For this review, take the finished solid that the model builds, in its own axes (mm). A direction names the side the tool comes from. Round coordinates to 2 decimals unless told otherwise and drop trailing zeros. Order: outer loops, then holes, each group sorted by start corner. A loop starts at its lowest first (then second) coordinate and runs counter-clockwise, first axis right, second up. Notation, with made-up numbers: M -21,82 L -7,82 A18 ccw -7,91 Z; hole C -22,15 d1. An arc over 180 degrees is marked long. Answer in a Markdown table with one row per item. Add a question column.
```python
from build123d import *

# Parameters (mm, degrees)
SKETCH_1_W          = 1.5
SKETCH_1_H          = 3
SKETCH_1_W_2        = 3.5
EXTRUDE_1_DEPTH     = 7
SKETCH_2_R          = 1.5
CUT_EXTRUDE_2_DEPTH = 7
SKETCH_4_R          = 1.5
CUT_EXTRUDE_3_DEPTH = 7


with BuildPart() as part:
    # 草图1 → 凸台-拉伸1 (new body)
    with BuildSketch(Plane.XY):
        Polygon((-0.641080243, 21.986723194), (-3.641080243, 21.986723194), (-3.641080243, -9.013276806), (-10.005041274, -15.377237837), (-10.005041274, -31.619878524), (-4.341080243, -31.619878524), (-4.341080243, -28.619878524), (-7.005041274, -28.619878524), (-7.005041274, -16.619878524), (-0.641080243, -10.255917493), align=None)
        with Locations((-2.091080243, -30.119878524)):
            Rectangle(SKETCH_1_W, SKETCH_1_H)
        with Locations((-3.591080243, -30.119878524)):
            Rectangle(SKETCH_1_W, SKETCH_1_H)
        with Locations((0.408919757, -30.119878524)):
            Rectangle(SKETCH_1_W_2, SKETCH_1_H)
    extrude(amount=EXTRUDE_1_DEPTH)

    # 草图2 → 切除-拉伸2 (cut)
    with BuildSketch(Plane.ZY.offset(3.641080243)):
        with Locations(Location((3.5, 18.986723194, 0), (0, 0, 270))):
            Circle(SKETCH_2_R)
        with Locations(Location((3.5, -3.013276806, 0), (0, 0, 270))):
            Circle(SKETCH_2_R)
    extrude(amount=-CUT_EXTRUDE_2_DEPTH, mode=Mode.SUBTRACT)

    # 草图4 → 切除-拉伸3 (cut)
    with BuildSketch(Plane(origin=(0, -28.619878524, 0), x_dir=(1, 0, 0), z_dir=(0, 1, 0))):
        with Locations(Location((-2.841080243, -4, 0), (0, 0, 270))):
            Circle(SKETCH_4_R)
    extrude(amount=-CUT_EXTRUDE_3_DEPTH, mode=Mode.SUBTRACT)


solid = part.part
```
1. The part is to be moulded in two halves that separate along Z. For faces 1 (the cylindrical face through (-3.416, -30.099, 5.386)), 2 (the cylindrical face through (-2.16, -3.71, 2.17)), 3 (the flat face through (-3, -7, 0)), 4 (the flat face through (-10.005, -23, 3)), say which applies: pulls with the +Z half, pulls with the -Z half, needs draft (parallel to the pull), parting line crosses it, or undercut.
2. Clearance check with flat-ended pins moving along their axes: pin 1 Ø1 at (y, z) = (-10, 3) entering from +X; pin 2 Ø2.5 at (y, z) = (-3.01, 3.5) entering from +X; pin 3 Ø2 at (x, z) = (-6, 3.5) entering from +Y. State where each tip first meets the part, or that it passes through.
3. Consider section D-D on x = 0.5. Write out the cut boundary in (y, z).
4. Consider section B-B on x = -2.25. Write out the cut boundary in (y, z), plus the area to 3 significant figures.
5. Consider section C-C on y = 17. Write out the cut boundary in (x, z), plus the area to 3 significant figures.
6. To check wall thickness, follow probe 1 along X at (y, z) = (-30.05, 4); probe 2 along X at (y, z) = (-20.5, 3); probe 3 along Y at (x, z) = (1, 5). State the ranges of each line that lie inside material, in increasing order. Write a range as [from, to].
7. Consider section A-A on z = 3. Write out the cut boundary in (x, y), plus the area to 3 significant figures.
8. For faces 5 (the flat face through (2.159, -30, 3)), 6 (the flat face through (-0.641, 6, 3)), 7 (the flat face through (-3.868, -13.482, 3.451)), 8 (the flat face through (-3.641, 7, 3)), list the 3-axis set-ups (+Z, -Z, +X, -X, +Y, -Y) from which the entire face can be reached by the end or side of a thin tool; tool diameter is ignored.
Solved:
| question | item | result |
|---|---|---|
| 1 | face 1 | undercut |
| 1 | face 2 | undercut |
| 1 | face 3 | pulls with the -Z half |
| 1 | face 4 | needs draft |
| 2 | pin 1 | stops at x = -0.64 |
| 2 | pin 2 | passes through |
| 2 | pin 3 | stops at y = -10.37 |
| 3 | outline | M -31.62,0 L -28.62,0 L -28.62,7 L -31.62,7 Z |
| 4 | outline | M -31.62,0 L -28.62,0 L -28.62,2.62 L -31.62,2.62 Z; M -31.62,5.38 L -28.62,5.38 L -28.62,7 L -31.62,7 Z; M -11.86,0 L 21.99,0 L 21.99,7 L -11.86,7 Z; hole C -3.01,3.5 d3; hole C 18.99,3.5 d3 |
| 4 | area | 236 mm^2 |
| 5 | outline | M -3.64,0 L -0.64,0 L -0.64,7 L -3.64,7 Z |
| 5 | area | 21.0 mm^2 |
| 6 | probe 1 | x = [-10.01, -4.34], [-1.34, 2.16] |
| 6 | probe 2 | x = [-10.01, -7.01] |
| 6 | probe 3 | y = [-31.62, -28.62] |
| 7 | outline | M -10.01,-31.62 L -3.96,-31.62 L -3.96,-28.62 L -7.01,-28.62 L -7.01,-16.62 L -0.64,-10.26 L -0.64,-4.43 L -3.64,-4.43 L -3.64,-9.01 L -10.01,-15.38 Z; M -3.64,-1.6 L -0.64,-1.6 L -0.64,17.57 L -3.64,17.57 Z; M -3.64,20.4 L -0.64,20.4 L -0.64,21.99 L -3.64,21.99 Z; M -1.72,-31.62 L 2.16,-31.62 L 2.16,-28.62 L -1.72,-28.62 Z |
| 7 | area | 173 mm^2 |
| 8 | face 5 | +Z, -Z, +X, +Y, -Y |
| 8 | face 6 | +Z, -Z, +X, +Y |
| 8 | face 7 | +Z, -Z, +X |
| 8 | face 8 | +Z, -Z, -X, +Y |
